Verification items for this drawing (mm, ordinates from the low corner). A direction names the side the tool comes from. Coordinates: 2 decimals unless noted, no trailing zeros. Loops run counter-clockwise (first coordinate to the right, second up) from the corner with the lowest first, then second, coordinate; pieces in that order, holes last. Notation, with made-up numbers: M -37.75,6 L 4.25,6 A23 ccw 4.25,31 Z; hole C 80.25,87.25 d10. An arc over 180 degrees is marked long. Write each question's results on one line, items separated by ' | '. Start each with the question number.
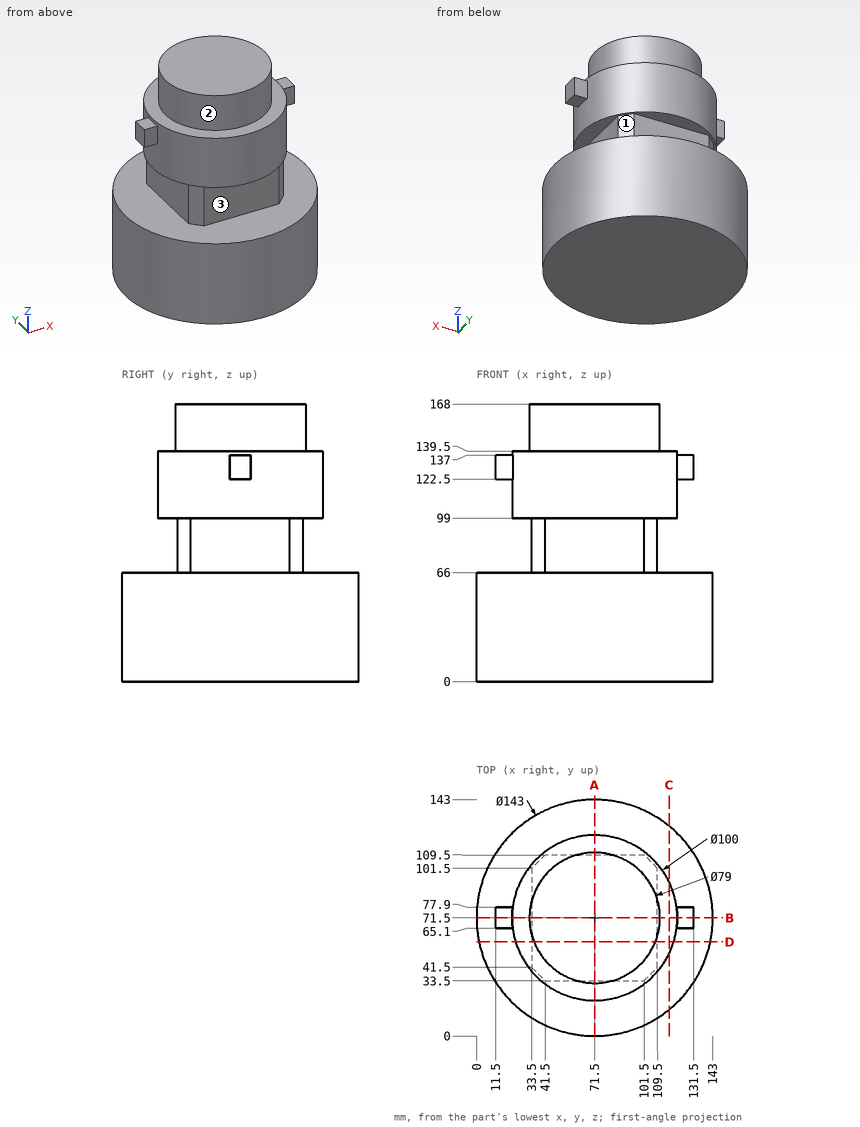
Item 1: Section check D-D (y = 57). Record the cut outline in (x, z), plus the area to 3 significant figures.
Item 2: Section check B-B (y = 71.5). Record the cut outline in (x, z), plus the area to 3 significant figures.
Item 3: Section check A-A (x = 71.5). Record the cut outline in (y, z).
Item 4: Tool access check on the marked faces 1, 2 and 3. Record the directions out of +Z, -Z, +X, -X, +Y, -Y that give a thin tool (end or side, any length) a straight path to the whole face; none if there is none.
Item 5: Depth check by flat-ended pin: P1, Ø3, axis at x = 18, z = 129, coming from the +Y side; P2, Ø3, axis at x = 125.5, y = 71.5, coming from the -Z side; P3, Ø10, axis at y = 77.5, z = 88.5, coming from the +X side; P4, Ø12, axis at y = 24.5, z = 24.5, coming from the +X side. Enter the tip coordinate at first touch or a pass-through.
Item 6: Thickness scan on line 1 (Z direction, x = 117, y = 58.5); line 2 (X direction, y = 73.5, z = 116); line 3 (X direction, y = 58, z = 76.5). Record the ranges inside material, lowest first.
Item 7: Section check C-C (x = 116.5). Record the cut outline in (y, z), plus the area to 3 significant figures.
Computed values:
1) outline: M 1.49,0 L 141.51,0 L 141.51,66 L 109.5,66 L 109.5,99 L 119.35,99 L 119.35,139.5 L 108.24,139.5 L 108.24,168 L 34.76,168 L 34.76,139.5 L 23.65,139.5 L 23.65,99 L 33.5,99 L 33.5,66 L 1.49,66 Z | area: 17,700 mm²
2) outline: M 0,0 L 143,0 L 143,66 L 109.5,66 L 109.5,99 L 121.5,99 L 121.5,122.5 L 131.5,122.5 L 131.5,137 L 121.5,137 L 121.5,139.5 L 111,139.5 L 111,168 L 32,168 L 32,139.5 L 21.5,139.5 L 21.5,137 L 11.5,137 L 11.5,122.5 L 21.5,122.5 L 21.5,99 L 33.5,99 L 33.5,66 L 0,66 Z | area: 18,500 mm²
3) outline: M 0,0 L 143,0 L 143,66 L 109.5,66 L 109.5,99 L 121.5,99 L 121.5,139.5 L 111,139.5 L 111,168 L 32,168 L 32,139.5 L 21.5,139.5 L 21.5,99 L 33.5,99 L 33.5,66 L 0,66 Z
4) face 1: +X, +Y | face 2: +Z | face 3: +X, -X, -Y
5) P1: stops at y = 77.9 | P2: stops at z = 0 | P3: stops at x = 109.5 | P4: stops at x = 130.08
6) line 1: z = 0 to 66, 99 to 139.5 | line 2: x = 21.54 to 121.46 | line 3: x = 33.5 to 109.5
7) outline: M 15.94,0 L 127.06,0 L 127.06,66 L 15.94,66 Z; M 49.71,99 L 93.29,99 L 93.29,139.5 L 49.71,139.5 Z | area: 9,100 mm²
